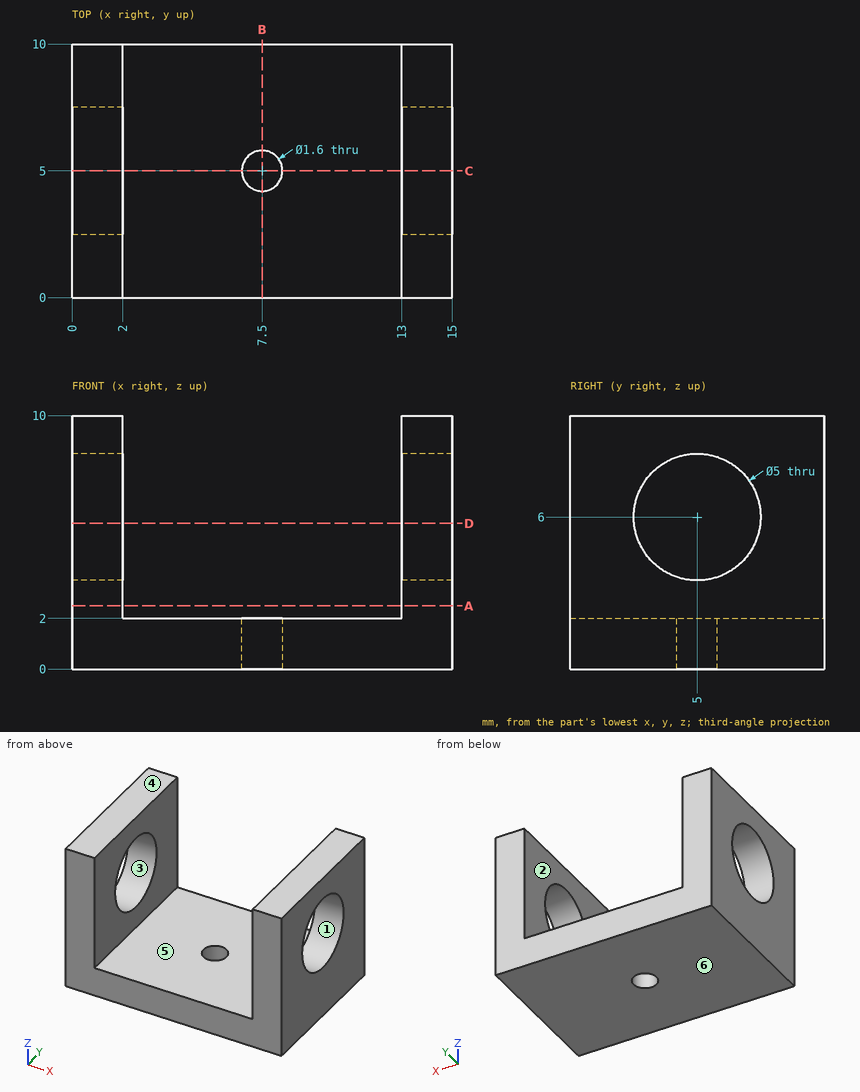
Answer from the drawing. Dimensions are ordinates in mm from the lowest x, y and z of the part. A direction names the side the tool comes from. Coordinates: 2 decimals unless noted, no trailing zeros. Write each loop counter-clockwise with the first axis right and the second up, starting at its lowest first coordinate (ties: lowest second). Pieces come first, ordered by that corner, then holes. Notation, with made-up numbers: M 26.5,25.5 L 62.5,25.5 A20 cw 62.5,54.5 Z; hole C 26.25,76.5 d1. An arc over 180 degrees is marked long. Use a Markdown table: item, result.
Q1. Each of these flat-tipped pins is pushed along its axis until it touches: pin 1 Ø1.8 at (x, y) = (7.5, 5) entering from +Z; pin 2 Ø3 at (y, z) = (5, 6) entering from +X. Where does it stop, or does it pass through?
Answer block:
| item | result |
|---|---|
| pin 1 | stops at z = 2 |
| pin 2 | passes through |
Q2. The part is cut by section D-D, the plane z = 5.75. Write down the section's boundary in (x, y), then the cut area to 3 significant figures.
Answer block:
| item | result |
|---|---|
| outline | M 0,0 L 2,0 L 2,2.51 L 0,2.51 Z; M 0,7.49 L 2,7.49 L 2,10 L 0,10 Z; M 13,0 L 15,0 L 15,2.51 L 13,2.51 Z; M 13,7.49 L 15,7.49 L 15,10 L 13,10 Z |
| area | 20.1 mm2 |
Q3. The part is cut by section C-C, the plane y = 5. Write down the section's boundary in (x, z), then the cut area to 3 significant figures.
Answer block:
| item | result |
|---|---|
| outline | M 0,0 L 6.7,0 L 6.7,2 L 2,2 L 2,3.5 L 0,3.5 Z; M 0,8.5 L 2,8.5 L 2,10 L 0,10 Z; M 8.3,0 L 15,0 L 15,3.5 L 13,3.5 L 13,2 L 8.3,2 Z; M 13,8.5 L 15,8.5 L 15,10 L 13,10 Z |
| area | 38.8 mm2 |
Q4. Straight lines are drawn through the part: L1, parallel to Z at x = 14.25, y = 5; L2, parallel to X at y = 7.25, z = 7.75; L3, parallel to Y at x = 7.5, z = 0.5. For each, find the intervals that lie inside material, in ascending order. Write a range as [from, to].
Answer block:
| item | result |
|---|---|
| L1 | z = [0, 3.5], [8.5, 10] |
| L2 | x = [0, 2], [13, 15] |
| L3 | y = [0, 4.2], [5.8, 10] |
Q5. Determine the mould class of the marked faces 1, 2, 3 and 4 for opening direction Z: released by +Z, released by -Z, zero draft, split by the parting line, or undercut.
Answer block:
| item | result |
|---|---|
| face 1 | undercut |
| face 2 | zero draft |
| face 3 | undercut |
| face 4 | released by +Z |
Q6. The part is cut by section A-A, the plane z = 2.5. Write down the section's boundary in (x, y), then the cut area to 3 significant figures.
Answer block:
| item | result |
|---|---|
| outline | M 0,0 L 2,0 L 2,10 L 0,10 Z; M 13,0 L 15,0 L 15,10 L 13,10 Z |
| area | 40.0 mm2 |
Q7. The part is cut by section B-B, the plane x = 7.5. Write down the section's boundary in (y, z).
Answer block:
| item | result |
|---|---|
| outline | M 0,0 L 4.2,0 L 4.2,2 L 0,2 Z; M 5.8,0 L 10,0 L 10,2 L 5.8,2 Z |
Q8. Which of the six approach directions +Z, -Z, +X, -X, +Y, -Y give full straight-line access (tool end or side, diameter ignored) to the marked faces 5 and 6?
Answer block:
| item | result |
|---|---|
| face 5 | +Z, +Y, -Y |
| face 6 | -Z, +X, -X, +Y, -Y |
